Here's how the part is built. I have some questions about the finished solid (model axes, mm). A direction names the side the tool comes from. Coordinates: 2 decimals unless noted, no trailing zeros. Write each loop counter-clockwise with the first axis right and the second up, starting at its lowest first coordinate (ties: lowest second). Pieces come first, ordered by that corner, then holes.
Autodesk Inventor part; units mm, degrees
ref_plane "YZ Plane" through (0, 0, 0) normal (1, 0, 0) x (0, 1, 0)
ref_plane "XZ Plane" through (0, 0, 0) normal (0, 1, 0) x (-1, 0, 0)
ref_plane "XY Plane" through (0, 0, 0) normal (0, 0, 1) x (1, 0, 0)
sketch "Sketch1" plane through (0, 0, 0) normal (0, 1, 0) x (-1, 0, 0)
  line L0 (0, 0) -> (82.55, 0)
  line L1 (82.55, 0) -> (82.55, -184.15)
  line L2 (82.55, -184.15) -> (0, -184.15)
  line L3 (0, -184.15) -> (0, 0)
  line L4 (88.9, -190.5) -> (88.9, 6.35)
  line L5 (88.9, 6.35) -> (-6.35, 6.35)
  line L6 (-6.35, 6.35) -> (-6.35, -190.5)
  line L7 (-6.35, -190.5) -> (88.9, -190.5)
  dimension "d0" = 184.15
  dimension "d1" = 82.55
  dimension "d2" = 6.35
extrude "Extrusion1" add sketch "Sketch1" along normal blind 6.35 contours L0 L1 L2 L3
extrude "Extrusion2" add sketch "Sketch1" along normal blind 152.4
sketch "Sketch2" plane through (-88.9, 0, -190.5) normal (-1, 0, 0) x (0, 0, 1)
  line L0 (53.0182, 127) -> (143.8318, 127)
  line L1 (143.8318, 127) -> (143.8318, 177.8)
  line L2 (143.8318, 177.8) -> (53.0182, 177.8)
  line L3 (53.0182, 177.8) -> (53.0182, 127)
  line L4 (190.5, 152.4) -> (6.35, 152.4)
  line L5 (53.0182, 127) -> (143.8318, 177.8) construction
  line L6 (143.8318, 127) -> (53.0182, 177.8) construction
  point P0 (190.5, 0)
  point P1 (98.425, 152.4)
  point P2 (53.0182, 152.4)
  point P3 (143.8318, 152.4)
  dimension "d14" = 25.4
extrude "Extrusion3" add sketch "Sketch2" against normal blind 6.35 contours L3 L2 L1 L4
fillet "Fillet1" radius 12.7 4 edges at (-85.725, 177.8, -46.6682) (-85.725, 152.4, -46.6682) (-85.725, 177.8, -137.4818) (-85.725, 152.4, -137.4818)
sketch "Sketch3" plane through (-82.55, 6.35, 0) normal (1, 0, 0) x (0, 0, -1)
  line L0 (124.7818, 171.45) -> (59.3682, 171.45)
  line L1 (92.075, 171.45) -> (92.075, 193.6256)
  line L2 (67.0657, 165.1) -> (117.0843, 165.1)
  line L3 (117.0843, 165.1) -> (117.0843, 160.109)
  line L4 (117.0843, 160.109) -> (67.0657, 160.109)
  line L5 (67.0657, 160.109) -> (67.0657, 165.1)
  line L6 (67.0657, 165.1) -> (117.0843, 160.109) construction
  line L7 (117.0843, 165.1) -> (67.0657, 160.109) construction
  point P0 (0, -6.35)
  point P1 (92.075, 162.6045)
  dimension "d15" = 6.35
extrude "Extrusion4" cut sketch "Sketch3" against normal blind 6.35
sketch "Sketch4" plane through (6.35, 0, 6.35) normal (1, 0, 0) x (0, 0, -1)
  line L0 (0, 152.4) -> (196.85, 152.4)
  line L1 (98.425, 152.4) -> (98.425, 129.719)
  circle A0 centre (98.425, 141.0595) radius 4.0936
  point P0 (6.35, 0)
extrude "Extrusion5" cut sketch "Sketch4" against normal up to surface (6.35 mm away)
sketch "Sketch5" plane through (6.35, 0, 6.35) normal (1, 0, 0) x (0, 0, -1)
  line L0 (196.85, 0) -> (196.85, 152.4)
  line L1 (0, 0) -> (196.85, 0)
  line L2 (196.85, 0) -> (196.85, 31.75)
  line L3 (196.85, 31.75) -> (0, 31.75)
  line L4 (0, 31.75) -> (0, 0)
  line L5 (0, 31.75) -> (62.6052, 31.75)
  line L6 (0, 31.75) -> (50.8, 31.75)
  line L7 (196.85, 31.75) -> (146.05, 31.75)
  circle A0 centre (50.8, 31.75) radius 2.0701
  circle A1 centre (146.05, 31.75) radius 2.0701
  point P0 (6.35, 0)
  dimension "d16" = 31.75
  dimension "d17" = 50.8
  dimension "d18" = 50.8
  dimension "d19" = 4.1402
  dimension "d20" = 4.1402
extrude "Extrusion6" cut sketch "Sketch5" against normal through all contours A1 L3 | L3 A1 | A0 L3 | L3 A0
properties material "Polycarbonate, Clear"
1) Imagine slicing it at A-A on z = -83. Please give me the cut outline in (x, y).
Values follow:
outline: (-88.9, 0) - (6.35, 0) - (6.35, 152.4) - (0, 152.4) - (0, 6.35) - (-82.55, 6.35) - (-82.55, 166.46) - (-88.9, 166.46) - close; (-88.9, 171.45) - (-82.55, 171.45) - (-82.55, 177.8) - (-88.9, 177.8) - close
2) We'd pull the mould along Y, two halves only. Please class faces 1 (the face through (-88.9, 88, -93)), 2 (the face through (-86, 169, -117.084)), 3 (the face through (1, 152.4, -92)): pulls with the +Y half, pulls with the -Y half, needs draft (parallel to the pull), parting line crosses it, or undercut.
Values follow:
face 1: needs draft
face 2: undercut
face 3: pulls with the +Y half
3) On a 3-axis mill with a long thin cutter (end or side, diameter ignored), from which of +Z, -Z, +X, -X, +Y, -Y can I reach the whole of each face in a straight line? I mean faces 4 (the face through (-42, 78, -184.15)), 5 (the face through (-86, 171.45, -92)), 6 (the face through (3.219, 141.239, -87.985)). Say none if no direction works.
Values follow:
face 4: +Y
face 5: +X, -X
face 6: +X
4) Imagine slicing it at C-C on z = -25. Please give me the cut outline in (x, y).
Values follow:
outline: (-88.9, 0) - (6.35, 0) - (6.35, 152.4) - (0, 152.4) - (0, 6.35) - (-82.55, 6.35) - (-82.55, 152.4) - (-88.9, 152.4) - close
5) I need wall thicknesses on probe 1 along Z at (x, y) = (3.5, 31.75); probe 2 along X at (y, z) = (145.5, -2); probe 3 along Z at (x, y) = (-33, 16). Which ranges of each line are inside material? Lowest first, please.
Values follow:
probe 1: z = -190.5 to -141.77, -137.63 to -46.52, -42.38 to 6.35
probe 2: x = -88.9 to -82.55, 0 to 6.35
probe 3: z = -190.5 to -184.15, 0 to 6.35
6) Imagine slicing it at B-B on y = 47. Please give me the cut outline in (x, z), then the cut area to 3 significant figures.
Values follow:
outline: (-88.9, -190.5) - (6.35, -190.5) - (6.35, 6.35) - (-88.9, 6.35) - close; hole (-82.55, -184.15) - (0, -184.15) - (0, 0) - (-82.55, 0) - close
area: 3,550 mm2
7) Imagine slicing it at D-D on x = -23. Please give me the cut outline in (y, z).
Values follow:
outline: (0, -190.5) - (152.4, -190.5) - (152.4, -184.15) - (6.35, -184.15) - (6.35, 0) - (152.4, 0) - (152.4, 6.35) - (0, 6.35) - close
8) Will these pins go through, and if not, where does the flat tip stop? pin 1 (7.5 mm diameter, centred on y = 141.06, z = -92.08, fed in from +X); pin 2 (10 mm diameter, centred on x = -41, z = -137.5, fed in from +Y).
Values follow:
pin 1: stops at x = -82.55
pin 2: stops at y = 6.35
